The drawing under review shows one solid part. Ordinate dimensions are in mm from its lowest x, y, z. Coordinates: 2 decimals unless noted, no trailing zeros. Write each loop counter-clockwise with the first axis right and the second up, starting at its lowest first coordinate (ties: lowest second). Pieces come first, ordered by that corner, then holes.
1) Mouldability with a two-part tool opening along Y and no side actions: class the marked faces 1 and 2 as released by +Y, released by -Y, zero draft, split by the parting line, or undercut.
2) Add section A-A, the plane z = 19.5. State the section outline as (x, y) points.
3) Add section D-D, the plane y = 1.35. Give the number of separate pieces and of enclosed holes in the cut face.
4) Add section B-B, the plane z = 14.5. State the section outline as (x, y) points (1 decimal).
5) Add section C-C, the plane x = 21.5. State the section outline as (y, z) points (1 decimal), then the cut area to 3 significant figures.
6) For line 1 (X direction, y = 0.8, z = 14.5) (1 decimal); line 2 (X direction, y = 1.25, z = 24.5) (1 decimal); line 3 (X direction, y = 1.2, z = 2.87) (1 decimal), list the stretches that pass through material, from the lowest coordinate up.
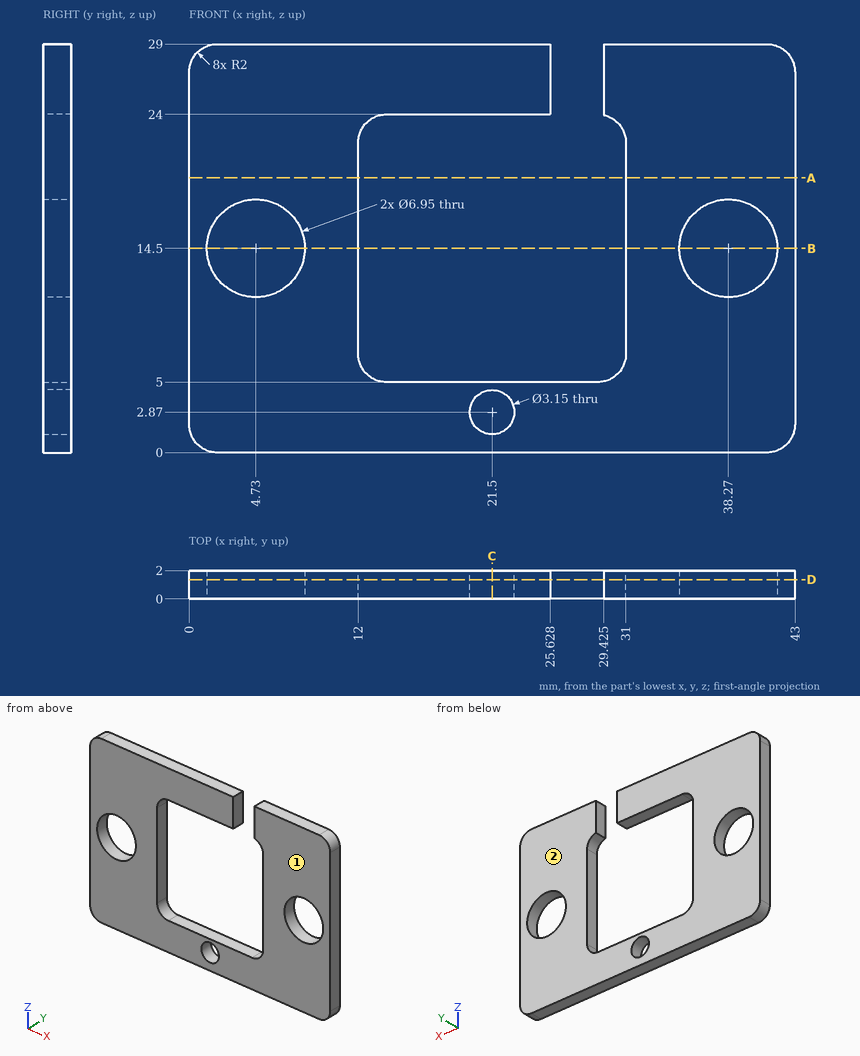
Geometry results:
1. face 1: released by -Y
1. face 2: released by +Y
2. outline: (0, 0) - (12, 0) - (12, 2) - (0, 2) - close; (31, 0) - (43, 0) - (43, 2) - (31, 2) - close
3. separate pieces: 1
3. enclosed holes: 3
4. outline: (0, 0) - (1.3, 0) - (1.3, 2) - (0, 2) - close; (8.2, 0) - (12, 0) - (12, 2) - (8.2, 2) - close; (31, 0) - (34.8, 0) - (34.8, 2) - (31, 2) - close; (41.7, 0) - (43, 0) - (43, 2) - (41.7, 2) - close
5. outline: (0, 0) - (2, 0) - (2, 1.3) - (0, 1.3) - close; (0, 4.4) - (2, 4.4) - (2, 5) - (0, 5) - close; (0, 24) - (2, 24) - (2, 29) - (0, 29) - close
5. area: 13.7 mm2
6. line 1: x = 0 to 1.3, 8.2 to 12, 31 to 34.8, 41.7 to 43
6. line 2: x = 0 to 25.6, 29.4 to 43
6. line 3: x = 0 to 19.9, 23.1 to 43
